from build123d import *

# Parameters (mm, degrees)
F0_W     = 140
F0_H     = 220
F1_DEPTH = 6
F3_D     = 4.1
F4_D     = 3.2
F2_R     = 19.05
F2_R_2   = 4
F2_R_3   = 6
F5_DEPTH = 6.001
F6_R     = 4
F8_D     = 3.2
F9_D     = 4.1


with BuildPart() as f1:
    # F0 (on Front) → F1 (new body)
    with BuildSketch(Plane.XZ):
        with Locations((0, 30)):
            Rectangle(F0_W, F0_H)
    extrude(amount=F1_DEPTH)

    # F3 (through all)
    with Locations(Plane.XZ.offset(6)):
        with Locations((-13.5, 66), (13.5, 66)):
            Hole(F3_D / 2)

    # F4 (through all)
    with Locations(Plane.XZ.offset(6)):
        with Locations((-23.55, 123.55), (23.55, 123.55), (23.55, 76.45), (-23.55, 76.45)):
            Hole(F4_D / 2)

    # F2 (on face) → F5 (cut, through all)
    with BuildSketch(Plane.XZ.offset(6)):
        with Locations((0, 100)):
            Circle(F2_R)
        with Locations((-55, 65)):
            Circle(F2_R_2)
        with Locations((55, 65)):
            Circle(F2_R_2)
        with Locations((-55, -65.3)):
            Circle(F2_R_3)
        with Locations((55, -65.3)):
            Circle(F2_R_3)
    extrude(amount=-F5_DEPTH, mode=Mode.SUBTRACT)

    # F6
    f6_edges = [f1.edges().sort_by_distance(p)[0] for p in [
        (70, -3, 140),
        (-70, -3, 140),
        (-70, -3, -80),
        (70, -3, -80),
    ]]
    fillet(f6_edges, radius=F6_R)

    # F8 (through all)
    with Locations(Plane.XZ.offset(6)):
        with Locations((-45, 20), (-45, 0), (-45, -20), (-25, -65), (25, -65), (45, -20), (45, 0), (45, 20), (0, 0)):
            Hole(F8_D / 2)

    # F9 (through all)
    with Locations(Plane.XZ.offset(6)):
        with Locations((-60, 130), (-60, 100), (60, 130), (60, 100), (-40, 130), (40, 130)):
            Hole(F9_D / 2)


solid = f1.part
The listing builds one solid part. Answer for the finished solid, in the listing's coordinates (mm). Coordinates: 2 decimals unless noted, no trailing zeros. Order: outer loops, then holes, each group sorted by start corner. A loop starts at its lowest first (then second) coordinate and runs counter-clockwise, first axis right, second up.
Q1. A cutting plane is placed at C-C, the plane z = 111. Write down the section's boundary in (x, y), and give its area (3 significant figures).
Q2. A cutting plane is placed at A-A, the plane y = -2.9. State how many separate pieces and enclosed holes the cut face has, and give its area (3 significant figures).
Q3. Given P1, Ø4, axis at x = -23.55, z = 123.55, coming from the -Y side, flat-ended and moving along its own axis, determine where the tip first touches the part or whether it passes through.
Q4. Consider line 1 (Z direction, x = -55, y = -5.65); line 2 (Z direction, x = 0, y = -1.35); line 3 (X direction, y = -1.3, z = -62.5). Determine where each line is inside the solid, lowest interval first.
Q5. A cutting plane is placed at B-B, the plane x = -55. Write down the section's boundary in (y, z), and give its area (3 significant figures).
Answers follow:
1. outline: (-70, -6) - (-15.55, -6) - (-15.55, 0) - (-70, 0) - close; (15.55, -6) - (70, -6) - (70, 0) - (15.55, 0) - close
1. area: 653 mm2
2. separate pieces: 1
2. enclosed holes: 26
2. area: 29,100 mm2
3. P1: stops at y = -6
4. line 1: z = -80 to -71.3, -59.3 to 61, 69 to 140
4. line 2: z = -80 to -1.6, 1.6 to 80.95, 119.05 to 140
4. line 3: x = -70 to -60.31, -49.69 to 49.69, 60.31 to 70
5. outline: (-6, -80) - (0, -80) - (0, -71.3) - (-6, -71.3) - close; (-6, -59.3) - (0, -59.3) - (0, 61) - (-6, 61) - close; (-6, 69) - (0, 69) - (0, 140) - (-6, 140) - close
5. area: 1,200 mm2
